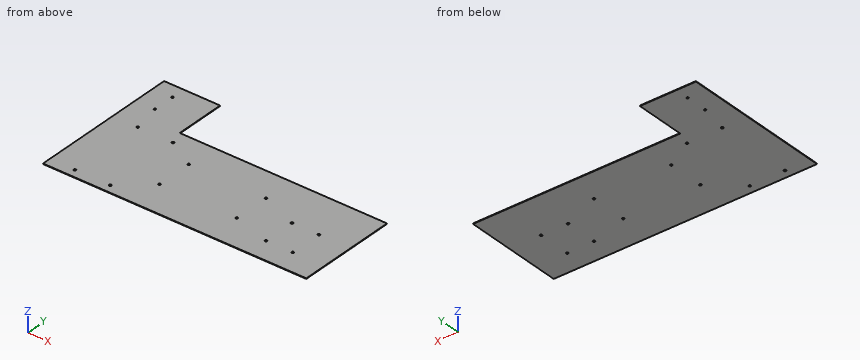
```python
from build123d import *

# Parameters (mm, degrees)
F1_DEPTH = 1
F2_R     = 2
F3_DEPTH = 1
F4_R     = 2
F5_DEPTH = 25
F6_R     = 2
F7_DEPTH = 25
F8_R     = 1.75
F9_DEPTH = 25


with BuildPart() as f1:
    # F0 (on Top) → F1 (new body)
    with BuildSketch(Plane.XY):
        Polygon((-235, 90), (-235, -90), (235, -90), (235, 90), (-135, 90), (-135, 180), (-235, 180), align=None)
    extrude(amount=F1_DEPTH)

    # F2 (on face) → F3 (cut, through all)
    with BuildSketch(Plane.XY.offset(1)):
        with Locations((-127, 65)):
            Circle(F2_R)
        with Locations((-190, 65)):
            Circle(F2_R)
        with Locations((-127, -75)):
            Circle(F2_R)
        with Locations((-190, -75)):
            Circle(F2_R)
    extrude(amount=-F3_DEPTH, mode=Mode.SUBTRACT)

    # F4 (on face) → F5 (cut)
    with BuildSketch(Plane.XY.offset(1)):
        with Locations((-75, 35)):
            Circle(F4_R)
        with Locations((63, 35)):
            Circle(F4_R)
        with Locations((-75, -30)):
            Circle(F4_R)
        with Locations((63, -30)):
            Circle(F4_R)
    extrude(amount=-F5_DEPTH, mode=Mode.SUBTRACT)

    # F6 (on face) → F7 (cut)
    with BuildSketch(Plane.XY.offset(1)):
        with Locations((131, 8)):
            Circle(F6_R)
        with Locations((131, -50)):
            Circle(F6_R)
        with Locations((179, 8)):
            Circle(F6_R)
        with Locations((179, -50)):
            Circle(F6_R)
    extrude(amount=-F7_DEPTH, mode=Mode.SUBTRACT)

    # F8 (on face) → F9 (cut)
    with BuildSketch(Plane.XY.offset(1)):
        with Locations((-200, 155)):
            Circle(F8_R)
        with Locations((-200, 115.9)):
            Circle(F8_R)
    extrude(amount=-F9_DEPTH, mode=Mode.SUBTRACT)


solid = f1.part
```
Model file for the job. Use its own axes, mm. Give positions to 0.01 mm unless a question says otherwise; leave off trailing zeros. Loops run counter-clockwise (first coordinate to the right, second up) from the corner with the lowest first, then second, coordinate; pieces in that order, holes last. Notation, with made-up numbers: (10, 67.25) -> (58, 67.25) arc R17 ccw to (58, 79.25) -> close; hole circle Ø9 at (46, -13). An arc over 180 degrees is marked (long way). Use CSV: the item, a comma, the result in double quotes. Start each with the question number.
1) Slice it at B-B on x = -54.5. Give the cut face in (y, z), plus the area to 3 significant figures.
2) Slice it at A-A on z = 0.85. Give the number of separate pieces and of enclosed holes in the cut face, plus the area to 3 significant figures.
3) Flat gauge pin, fed straight in: pin 1 Ø3.5 at (x, y) = (63, -30) entering from -Z. Where does the tip first touch, or does it go through?
4) Wall check: line 1 (Y direction, x = -127, z = 0.65); line 2 (Y direction, x = -200, z = 0.45); line 3 (Y direction, x = 88, z = 0.8). Give the ranges that are in metal, low to high.
Computed values:
1,outline,"(-90, 0) -> (90, 0) -> (90, 1) -> (-90, 1) -> close"
1,area,"180 mm^2"
2,separate pieces,"1"
2,enclosed holes,"14"
2,area,"93,400 mm^2"
3,pin 1,"passes through"
4,line 1,"y = -90 to -77, -73 to 63, 67 to 90"
4,line 2,"y = -90 to 114.15, 117.65 to 153.25, 156.75 to 180"
4,line 3,"y = -90 to 90"
